Build history of the part. All positions in model axes, mm. A direction names the side the tool comes from. Round coordinates to 2 decimals unless told otherwise and drop trailing zeros. Write each loop counter-clockwise with the first axis right and the second up, starting at its lowest first coordinate (ties: lowest second). Pieces come first, ordered by that corner, then holes. Notation, with made-up numbers: (60, 26) -> (85, 26) arc R22 cw to (85, 59) -> close; hole circle Ø9 at (16.25, -21.75). An arc over 180 degrees is marked (long way). Answer in a Markdown table with one row per item. Add a question column.
from build123d import *

# Parameters (mm, degrees)
F1_DEPTH = 10
F2_R     = 10
F3_DEPTH = 8


with BuildPart() as f1:
    # F0 (on Top) → F1 (new body)
    with BuildSketch(Plane.XY):
        with BuildLine():
            ThreePointArc((6, 0), (0, 6), (-6, 0))
            ThreePointArc((-6, 0), (0, -6), (6, 0))
        make_face()
        with BuildLine():
            ThreePointArc((0.720724, -17.985565), (12.980236, -12.470505), (18, 0))
            ThreePointArc((18, 0), (12.980236, 12.470505), (0.720724, 17.985565))
            ThreePointArc((0.720724, 17.985565), (-12.470505, 12.980236), (-18, 0))
            ThreePointArc((-18, 0), (-12.470505, -12.980236), (0.720724, -17.985565))
        make_face()
        with BuildLine():
            ThreePointArc((6, 0), (0, -6), (-6, 0))
            ThreePointArc((-6, 0), (0, 6), (6, 0))
        make_face(mode=Mode.SUBTRACT)
        with BuildLine():
            ThreePointArc((-18, 0), (-12.470505, 12.980236), (0.720724, 17.985565))
            ThreePointArc((0.720724, 17.985565), (-19.637945, 23.224109), (-36.043982, 36.367918))
            ThreePointArc((-36.043982, 36.367918), (-33.041104, 31.032896), (-32, 25))
            ThreePointArc((-32, 25), (-37.272078, 12.272078), (-50, 7))
            Line((-50, 7), (-50, 0))
            Line((-50, 0), (-18, 0))
        make_face()
        with BuildLine():
            ThreePointArc((-36.043982, -36.367918), (-19.637945, -23.224109), (0.720724, -17.985565))
            ThreePointArc((0.720724, -17.985565), (-12.470505, -12.980236), (-18, 0))
            Line((-18, 0), (-50, 0))
            Line((-50, 0), (-50, -7))
            ThreePointArc((-50, -7), (-37.272078, -12.272078), (-32, -25))
            ThreePointArc((-32, -25), (-33.041104, -31.032896), (-36.043982, -36.367918))
        make_face()
        with BuildLine():
            ThreePointArc((-44, 25), (-54.242641, 29.242641), (-50, 19))
            ThreePointArc((-50, 19), (-45.757359, 20.757359), (-44, 25))
        make_face()
        with BuildLine():
            ThreePointArc((-32, 25), (-33.041104, 31.032896), (-36.043982, 36.367918))
            ThreePointArc((-36.043982, 36.367918), (-56.308566, 41.858292), (-67.990432, 24.413191))
            ThreePointArc((-67.990432, 24.413191), (-62.518735, 12.066273), (-50, 7))
            ThreePointArc((-50, 7), (-37.272078, 12.272078), (-32, 25))
        make_face()
        with BuildLine():
            ThreePointArc((-44, 25), (-45.757359, 20.757359), (-50, 19))
            ThreePointArc((-50, 19), (-54.242641, 29.242641), (-44, 25))
        make_face(mode=Mode.SUBTRACT)
        with BuildLine():
            ThreePointArc((-44, -25), (-45.757359, -20.757359), (-50, -19))
            ThreePointArc((-50, -19), (-54.242641, -29.242641), (-44, -25))
        make_face()
        with BuildLine():
            ThreePointArc((-67.990432, -25.586809), (-55.755624, -42.054993), (-36.043982, -36.367918))
            ThreePointArc((-36.043982, -36.367918), (-33.041104, -31.032896), (-32, -25))
            ThreePointArc((-32, -25), (-37.272078, -12.272078), (-50, -7))
            ThreePointArc((-50, -7), (-62.518735, -12.066273), (-67.990432, -24.413191))
            Line((-67.990432, -24.413191), (-67.990432, -25.586809))
        make_face()
        with BuildLine():
            ThreePointArc((-44, -25), (-54.242641, -29.242641), (-50, -19))
            ThreePointArc((-50, -19), (-45.757359, -20.757359), (-44, -25))
        make_face(mode=Mode.SUBTRACT)
        with BuildLine():
            Line((-50, -7), (-50, 0))
            Line((-50, 0), (-50, 7))
            ThreePointArc((-50, 7), (-62.518735, 12.066273), (-67.990432, 24.413191))
            Line((-67.990432, 24.413191), (-67.990432, -24.413191))
            ThreePointArc((-67.990432, -24.413191), (-62.518735, -12.066273), (-50, -7))
        make_face()
        with BuildLine():
            ThreePointArc((-67.990432, -24.413191), (-68, -25), (-67.990432, -25.586809))
            Line((-67.990432, -25.586809), (-67.990432, -24.413191))
        make_face()
    extrude(amount=F1_DEPTH)

    # F2 (on Front) → F3 (join, symmetric)
    with BuildSketch(Plane.XZ):
        with BuildLine():
            ThreePointArc((-110, 0), (-94.443651, 6.443651), (-88, 22))
            ThreePointArc((-88, 22), (-90.080579, 31.338987), (-95.928789, 38.911565))
            ThreePointArc((-95.928789, 38.911565), (-130.688818, 29.481496), (-110, 0))
        make_face()
        with Locations((-110, 22)):
            Circle(F2_R, mode=Mode.SUBTRACT)
        with BuildLine():
            ThreePointArc((-95.928789, 38.911565), (-90.080579, 31.338987), (-88, 22))
            ThreePointArc((-88, 22), (-94.443651, 6.443651), (-110, 0))
            Line((-110, 0), (-15.978726, 0))
            Line((-15.978726, 0), (-15.978726, 10))
            ThreePointArc((-15.978726, 10), (-58.487228, 17.449895), (-95.928789, 38.911565))
        make_face()
    extrude(amount=F3_DEPTH, both=True)


solid = f1.part
(1) Probe line 1 along Y through (x, z) = (-50, 5.5); line 2 along Z through (x, y) = (-16, -17.5); line 3 along X through (y, z) = (-25, 5). List the from-to ranges inside material, lowest first.
(2) Drop flat-ended pins along their axis: P1, Ø22, axis at x = -70.5, z = 32, coming from the -Y side; P2, Ø18, axis at x = -110, z = 22, coming from the -Y side; P3, Ø11, axis at y = -14.5, z = 2.5, coming from the -X side; P4, Ø4, axis at y = -25.5, z = 7.5, coming from the +X side. Give the stop position or say it passes through.
(3) Saw through at D-D (x = -39.5). List the corners of the cut face in (y, z).
(4) Saw through at A-A (z = 22). List the corners of the cut face in (x, y), plus the area to 3 significant figures.
(5) Which spindle directions (+Z, -Z, +X, -X, +Y, -Y) get a long thin tool onto all of the face, cutting with end or side? Do faces 5 (the face through (-56.044, -41.955, 4.93)), 6 (the face through (-67.99, -16, 5)). Say none if no direction does.
(6) Saw through at C-C (z = 3). List the corners of the cut face in (x, y).
(7) Mould opens along X. For faces 1 (the face through (-130.481, -0.112, 30.034)), 2 (the face through (-117.37, 0.11, 28.76)), 3 (the face through (6, 0, 5)), 4 (the face through (-67.99, 16, 5)) say: pulls with the +X half, pulls with the -X half, needs draft (parallel to the pull), parting line crosses it, or undercut.
(8) Saw through at B-B (x = -117). List the corners of the cut face in (y, z).
Answer sheet:
| question | item | result |
|---|---|---|
| 1 | line 1 | y = -43 to -31, -19 to 19, 31 to 43 |
| 1 | line 2 | z = 0 to 10 |
| 1 | line 3 | x = -68 to -56, -44 to -22.88 |
| 2 | P1 | stops at y = -8 |
| 2 | P2 | passes through |
| 2 | P3 | stops at x = -67.99 |
| 2 | P4 | stops at x = -20.18 |
| 3 | outline | (-39.62, 0) -> (39.62, 0) -> (39.62, 10) -> (8, 10) -> (8, 12.23) -> (-8, 12.23) -> (-8, 10) -> (-39.62, 10) -> close |
| 4 | outline | (-132, -8) -> (-120, -8) -> (-120, 8) -> (-132, 8) -> close; (-100, -8) -> (-69.42, -8) -> (-69.42, 8) -> (-100, 8) -> close |
| 4 | area | 681 mm² |
| 5 | face 5 | +Z, -Z, -Y |
| 5 | face 6 | +Z, -Z, -X, -Y |
| 6 | outline | (-121.09, -8) -> (-67.99, -8) -> (-67.99, -24.41) arc R18 ccw to (-67.99, -25.59) arc R18 ccw to (-36.04, -36.37) arc R50 cw to (0.72, -17.99) arc R18 ccw to (18, 0) arc R18 ccw to (0.72, 17.99) arc R50 cw to (-36.04, 36.37) arc R18 ccw to (-67.99, 24.41) -> (-67.99, 8) -> (-121.09, 8) -> close; hole (-50, -19) arc R6 ccw (long way) to (-44, -25) arc R6 ccw to start; hole (-50, 19) arc R6 ccw to (-44, 25) arc R6 ccw (long way) to start; hole circle Ø12 at (0, 0) |
| 7 | face 1 | parting line crosses it |
| 7 | face 2 | undercut |
| 7 | face 3 | undercut |
| 7 | face 4 | pulls with the -X half |
| 8 | outline | (-8, 1.14) -> (8, 1.14) -> (8, 14.86) -> (-8, 14.86) -> close; (-8, 29.14) -> (8, 29.14) -> (8, 42.86) -> (-8, 42.86) -> close |
